Part model, mm, in its own coordinate system. Round coordinates to 2 decimals unless told otherwise and drop trailing zeros. Loops run counter-clockwise (first coordinate to the right, second up) from the corner with the lowest first, then second, coordinate; pieces in that order, holes last. Notation, with made-up numbers: M -37,87.5 L -10,87.5 A13 cw -10,93.5 Z; hole C 33.25,65 d10. An arc over 180 degrees is marked long. Answer as CSV lines item,"result". Start each with the question number.
Item 1: Band-saw the part on C-C (x = -11). Give the cut face in (y, z), and give its area (3 significant figures).
Item 2: Band-saw the part on B-B (y = 1.5). Count the separate pieces of the cut face and the enclosed holes in it, and give its area (3 significant figures).
Item 3: Band-saw the part on D-D (z = -26.5). Give the cut face in (x, y), and give its area (3 significant figures).
Item 4: Band-saw the part on A-A (z = 0). Give the cut face in (x, y).
Item 5: Drop flat-ended pins along their axis: pin 1 Ø4 at (y, z) = (2.5, 4) entering from +X; pin 2 Ø6.5 at (x, z) = (-59.5, 63) entering from +Y. Give the stop position or say it passes through.
Item 6: Wall check: line 1 (X direction, y = 5.5, z = 1.5); line 2 (Z direction, x = -11, y = 0.5); line 3 (X direction, y = 4, z = 45.5). Give the ranges that are in metal, low to high.
```python
from build123d import *

# Parameters (mm, degrees)
RESSALTO_EXTRUS_O1_DEPTH                = 7
CASCA1_DEPTH                            = 7
FURO_ROSCADO_PARA_CONDU_TE_DE_M3X0_51_D = 3.15
CORTE_EXTRUS_O1_DEPTH                   = 124.517933921
CORTE_EXTRUS_O2_DEPTH                   = 3


# Read off the part's stored shape, not the designer's step: Casca1
with BuildPart() as part:
    # Esboço1 → Ressalto-extrusão1 (new body)
    with BuildSketch(Plane(origin=(0, 0, 0), x_dir=(1, 0, 0), z_dir=(0, 1, 0))):
        with BuildLine():
            Line((-37, -78.961003033), (37, -78.961003033))
            ThreePointArc((37, -78.961003033), (46.963540288, -73.472892169), (56.127920845, -66.734522563))
            Line((56.127920845, -66.734522563), (66.734522563, -56.127920845))
            ThreePointArc((66.734522563, -56.127920845), (87.2, 0), (66.734522563, 56.127920845))
            Line((66.734522563, 56.127920845), (56.127920845, 66.734522563))
            ThreePointArc((56.127920845, 66.734522563), (0, 87.2), (-56.127920845, 66.734522563))
            Line((-56.127920845, 66.734522563), (-66.734522563, 56.127920845))
            ThreePointArc((-66.734522563, 56.127920845), (-87.2, 0), (-66.734522563, -56.127920845))
            Line((-66.734522563, -56.127920845), (-56.127920845, -66.734522563))
            ThreePointArc((-56.127920845, -66.734522563), (-46.963540288, -73.472892169), (-37, -78.961003033))
        make_face()
    extrude(amount=RESSALTO_EXTRUS_O1_DEPTH)

    # Casca1 outline → Casca1 (cut)
    with BuildSketch(Plane(origin=(0, 0, 0), x_dir=(1, 0, 0), z_dir=(0, 1, 0))):
        with BuildLine():
            ThreePointArc((-57.870105501, 48.021775158), (-75.2, 0), (-57.870105501, -48.021775158))
            Line((-57.870105501, -48.021775158), (-48.021775158, -57.870105501))
            ThreePointArc((-48.021775158, -57.870105501), (-41.373205231, -62.795683681), (-34.223735518, -66.961003033))
            Line((-34.223735518, -66.961003033), (34.223735518, -66.961003033))
            ThreePointArc((34.223735518, -66.961003033), (41.373205231, -62.795683681), (48.021775158, -57.870105501))
            Line((48.021775158, -57.870105501), (57.870105501, -48.021775158))
            ThreePointArc((57.870105501, -48.021775158), (75.2, 0), (57.870105501, 48.021775158))
            Line((57.870105501, 48.021775158), (48.021775158, 57.870105501))
            ThreePointArc((48.021775158, 57.870105501), (0, 75.2), (-48.021775158, 57.870105501))
            Line((-48.021775158, 57.870105501), (-57.870105501, 48.021775158))
        make_face()
    extrude(amount=CASCA1_DEPTH, mode=Mode.SUBTRACT)

    # Furo roscado para conduíte de M3x0.51 (through all)
    with Locations(Plane(origin=(0, 7, 0), x_dir=(1, 0, 0), z_dir=(0, 1, 0))):
        with Locations((-27.361611466, 75.175409663), (-47.022820183, -64.72135955), (47.022820183, -64.72135955), (27.361611466, 75.175409663), (-65.532163543, -45.886114908), (-45.886114908, 65.532163543), (65.532163543, -45.886114908), (45.886114908, 65.532163543)):
            Hole(FURO_ROSCADO_PARA_CONDU_TE_DE_M3X0_51_D / 2)

    # Esboço5 → Corte-extrusão1 (cut, through all)
    with BuildSketch(Plane(origin=(0, 7, 0), x_dir=(1, 0, 0), z_dir=(0, 1, 0))):
        with BuildLine():
            Line((-24.644524413, 83.645008318), (-21.253076099, 72.134227357))
            ThreePointArc((-21.253076099, 72.134227357), (0, 75.2), (21.253076099, 72.134227357))
            Line((21.253076099, 72.134227357), (24.644524413, 83.645008318))
            ThreePointArc((24.644524413, 83.645008318), (0, 87.2), (-24.644524413, 83.645008318))
        make_face()
    extrude(amount=-CORTE_EXTRUS_O1_DEPTH, mode=Mode.SUBTRACT)

    # Esboço8 → Corte-extrusão2 (cut)
    with BuildSketch(Plane(origin=(0, 7, 0), x_dir=(1, 0, 0), z_dir=(0, 1, 0))):
        Polygon((-66.734522563, -56.127920845), (-63.906095438, -53.29949372), (-53.29949372, -63.906095438), (-56.127920845, -66.734522563), align=None)
        Polygon((-56.127920845, 66.734522563), (-53.29949372, 63.906095438), (-63.906095438, 53.29949372), (-66.734522563, 56.127920845), align=None)
        Polygon((66.734522563, -56.127920845), (63.906095438, -53.29949372), (53.29949372, -63.906095438), (56.127920845, -66.734522563), align=None)
        Polygon((66.734522563, 56.127920845), (63.906095438, 53.29949372), (53.29949372, 63.906095438), (56.127920845, 66.734522563), align=None)
    extrude(amount=-CORTE_EXTRUS_O2_DEPTH, mode=Mode.SUBTRACT)


solid = part.part
```
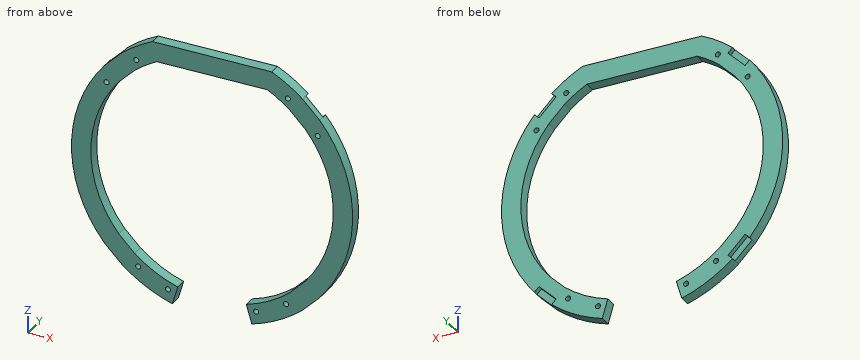
Answer block:
1,outline,"M 0,66.96 L 7,66.96 L 7,78.96 L 0,78.96 Z"
1,area,"84.0 mm^2"
2,separate pieces,"1"
2,enclosed holes,"8"
2,area,"5,470 mm^2"
3,outline,"M -83.08,0 L -70.38,0 L -70.38,7 L -83.08,7 Z; M 70.38,0 L 83.08,0 L 83.08,7 L 70.38,7 Z"
3,area,"178 mm^2"
4,outline,"M -87.2,0 L -75.2,0 L -75.2,7 L -87.2,7 Z; M 75.2,0 L 87.2,0 L 87.2,7 L 75.2,7 Z"
5,pin 1,"stops at x = 87.18"
5,pin 2,"stops at y = 4"
6,line 1,"x = -87.19 to -75.19, 75.19 to 87.19"
6,line 2,"z = 66.96 to 78.96"
6,line 3,"x = -74.39 to -67.06, -64.01 to -59.87, 59.87 to 64.01, 67.06 to 74.39"
